Geometry: final body of the model. Coordinates: model frame, mm. A direction names the side the tool comes from. Coordinates: 2 decimals unless noted, no trailing zeros. Write each loop counter-clockwise with the first axis right and the second up, starting at its lowest first coordinate (ties: lowest second). Pieces come first, ordered by that corner, then holes. Notation, with made-up numbers: (80, -31.75) - (84, -31.75) arc R4 cw to (84, -25.75) - close; hole circle Ø9 at (13.5, -10). An arc over 180 degrees is marked (long way). Answer as a JSON object with one key per item and string values. Group by question number.
Item 1: Section A-A on z = 61. Return loops of the section in (x, y), and give its area (4 significant figures).
Item 2: Mould query, pull axis Z, two halves, no side actions, for faces 3 (the flat face through (85, -9, 0)), 4 (the flat face through (176.53, -6, 44)), 5 (the flat face through (84, -6, -5.08)). Classes: pulls with the +Z half, pulls with the -Z half, needs draft (parallel to the pull), parting line crosses it, or undercut.
Item 3: Line query: line 1 along Z through (x, y) = (82, -7); line 2 along X through (y, z) = (-9.75, 17); line 3 along Y through (x, z) = (85, 85). Output: solid intervals per line, ascending. Write a range as from..to.
Item 4: Section C-C on x = 27. Return loops of the section in (y, z), and give its area (3 significant figures).
Item 5: Set-up query: faces 1 (the flat face through (85, -5.08, 45)), 2 (the flat face through (87, -6, 93.98)). Return all of +Z, -Z, +X, -X, +Y, -Y with unobstructed straight access to the full face (end or side cutting, diameter ignored); none if empty.
Item 6: Section B-B on y = -8.25. Return loops of the section in (x, z), and give its area (3 significant figures).
```python
from build123d import *

# Parameters (mm, degrees)
F0_W     = 171.45
F0_H     = 5.08
F1_DEPTH = 12.7
F0_H_2   = 88.9
F2_DEPTH = 5.08


with BuildPart() as f1:
    # F0 (on Front) → F1 (new body)
    with BuildSketch(Plane.XZ):
        Polygon((0, -5.08), (0, 0), (0, 88.9), (0, 93.98), (-5.08, 93.98), (-5.08, -5.08), align=None)
        with Locations((85.725, -2.54)):
            Rectangle(F0_W, F0_H)
        Polygon((171.45, 88.9), (171.45, 0), (171.45, -5.08), (176.53, -5.08), (176.53, 88.9), align=None)
        Polygon((0, 93.98), (0, 88.9), (171.45, 88.9), (176.53, 88.9), (176.53, 93.98), align=None)
    extrude(amount=F1_DEPTH)

    # F0 (on Front) → F2 (join)
    with BuildSketch(Plane.XZ):
        with Locations((85.725, 44.45)):
            Rectangle(F0_W, F0_H_2)
    extrude(amount=F2_DEPTH)


solid = f1.part
```
Checks:
{
 "1": {"outline": "(-5.08, -12.7) - (0, -12.7) - (0, -5.08) - (171.45, -5.08) - (171.45, -12.7) - (176.53, -12.7) - (176.53, 0) - (-5.08, 0) - close", "area": "1,000 mm^2"},
 "2": {"face 3": "undercut", "face 4": "needs draft", "face 5": "pulls with the -Z half"},
 "3": {"line 1": "-5.08..0, 88.9..93.98", "line 2": "-5.08..0, 171.45..176.53", "line 3": "-5.08..0"},
 "4": {"outline": "(-12.7, -5.08) - (0, -5.08) - (0, 93.98) - (-12.7, 93.98) - (-12.7, 88.9) - (-5.08, 88.9) - (-5.08, 0) - (-12.7, 0) - close", "area": "581 mm^2"},
 "5": {"face 1": "-Y", "face 2": "+Z, +X, -X, +Y, -Y"},
 "6": {"outline": "(-5.08, -5.08) - (176.53, -5.08) - (176.53, 93.98) - (-5.08, 93.98) - close; hole (0, 0) - (171.45, 0) - (171.45, 88.9) - (0, 88.9) - close", "area": "2,750 mm^2"}
}
